Read the model definition and answer for the solid it produces. Units are mm, in the model's axes. Coordinates: 2 decimals unless noted, no trailing zeros. Write each loop counter-clockwise with the first axis right and the second up, starting at its lowest first coordinate (ties: lowest second). Pieces come first, ordered by that corner, then holes. Notation, with made-up numbers: (-30.75, 58) -> (0.25, 58) arc R23 ccw to (0.25, 89) -> close; hole circle Ø10 at (53.5, -24). An arc over 180 degrees is marked (long way). Write item = value, one per line. Start each with the question number.
1) Section A-A (x = -114.3) is taken. Determine the outline of the cut face in (y, z) (1 decimal), plus the area to 3 significant figures.
2) A flat-ended cylindrical pin translates along its axis: pin 1 Ø3.5 at (x, z) = (-12.7, 12.7) entering from +Y (3 decimals). Find the tip coordinate at first contact, or state that the pin passes through.
3) Section B-B (x = -12.7) is taken. Determine the outline of the cut face in (y, z) (1 decimal).
4) Find the intervals of material crossed by line 1 along X through (y, z) = (0.95, 165.1); line 2 along X through (y, z) = (1, 140); line 3 along Z through (x, y) = (-101.6, 0.8), in increasing order. Write a range as from..to.
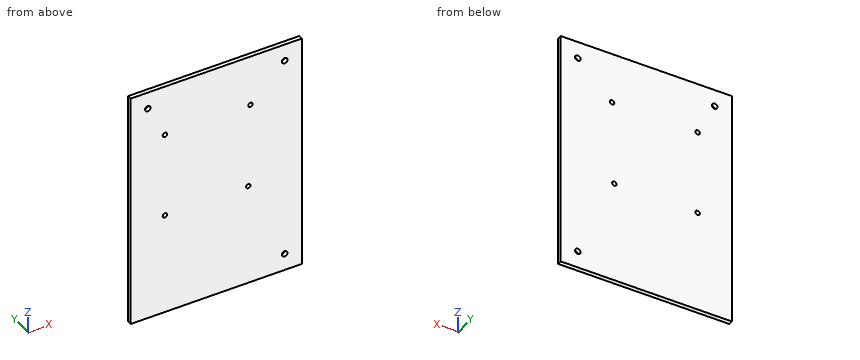
Autodesk Inventor part; units mm, degrees
ref_plane "YZ Plane" through (0, 0, 0) normal (1, 0, 0) x (0, 1, 0)
ref_plane "XZ Plane" through (0, 0, 0) normal (0, 1, 0) x (-1, 0, 0)
ref_plane "XY Plane" through (0, 0, 0) normal (0, 0, 1) x (1, 0, 0)
sketch "Base" plane through (0, 0, 0) normal (0, 1, 0) x (-1, 0, 0)
  line L0 (0, 0) -> (127, 0)
  line L1 (127, 0) -> (127, 177.8)
  line L2 (127, 177.8) -> (0, 177.8)
  line L3 (0, 177.8) -> (0, 0)
  dimension "d7" = 127
  dimension "d8" = 177.8
extrude "Base 1/8\"" add sketch "Base" along normal blind 3.175
sketch "TopLayer" plane through (0, 3.175, 0) normal (0, 1, 0) x (1, 0, 0)
  point P0 (-114.3, -165.1)
  point P1 (-12.7, -165.1)
  point P2 (-12.7, -12.7)
hole "TopLayerHoles" at (-114.3, 3.175, 165.1) at (-12.7, 3.175, 165.1) at (-12.7, 3.175, 12.7) direction (0, -1, 0) diameter 4.191 end through all
sketch "Controller" plane through (0, 3.175, 0) normal (0, 1, 0) x (1, 0, 0)
  line L0 (0, 0) -> (-127, 0)
  line L1 (-127, 0) -> (-127, -177.8)
  line L2 (-127, -152.4) -> (-25.4, -152.4) construction
  line L3 (-127, -152.4) -> (-25.4, -152.4) construction
  line L4 (-25.4, -152.4) -> (-25.4, 0) construction
  line L5 (-140.6178, -177.8) -> (-108.8678, -177.8) construction
  line L6 (-31.75, -146.05) -> (-107.95, -146.05) construction
  line L7 (-107.95, -146.05) -> (-107.95, -69.85) construction
  line L8 (-107.95, -69.85) -> (-31.75, -69.85) construction
  line L9 (-31.75, -69.85) -> (-31.75, -146.05) construction
  line L10 (-31.75, -146.05) -> (-38.1, -146.05) construction
  line L11 (-38.1, -146.05) -> (-38.1, -139.7) construction
  line L12 (-38.1, -139.7) -> (-31.75, -139.7) construction
  line L13 (-31.75, -139.7) -> (-31.75, -146.05) construction
  line L14 (-107.95, -69.85) -> (-101.6, -69.85) construction
  line L15 (-101.6, -69.85) -> (-101.6, -76.2) construction
  line L16 (-101.6, -76.2) -> (-107.95, -76.2) construction
  line L17 (-107.95, -76.2) -> (-107.95, -69.85) construction
  circle A0 centre (-38.1, -139.7) radius 1.651
  circle A1 centre (-101.6, -139.7) radius 1.651
  circle A2 centre (-101.6, -76.2) radius 1.651
  circle A3 centre (-39.751, -76.2) radius 1.651
  dimension "d36" = 76.2
  dimension "d37" = 76.2
  dimension "d38" = 6.35
  dimension "d39" = 6.35
  dimension "d40" = 6.35
  dimension "d41" = 6.35
  dimension "d42" = 3.302
  dimension "d43" = 3.302
  dimension "d44" = 3.302
  dimension "d45" = 3.302
hole "ControllerHoles" at (-38.1, 3.175, 139.7) at (-39.751, 3.175, 76.2) at (-101.6, 3.175, 76.2) at (-101.6, 3.175, 139.7) direction (0, -1, 0) diameter 3.302 end through all
properties part number "bottomLayer"
Answer key:
q1.outline = (0, 0) -> (3.2, 0) -> (3.2, 163) -> (0, 163) -> close; (0, 167.2) -> (3.2, 167.2) -> (3.2, 177.8) -> (0, 177.8) -> close
q1.area = 551 mm^2
q2.pin_1 = through
q3.outline = (0, 0) -> (3.2, 0) -> (3.2, 10.6) -> (0, 10.6) -> close; (0, 14.8) -> (3.2, 14.8) -> (3.2, 163) -> (0, 163) -> close; (0, 167.2) -> (3.2, 167.2) -> (3.2, 177.8) -> (0, 177.8) -> close
q4.line_1 = -127..-116.4, -112.2..-14.8, -10.6..0
q4.line_2 = -127..-103.22, -99.98..-39.72, -36.48..0
q4.line_3 = 0..74.55, 77.85..138.05, 141.35..177.8
